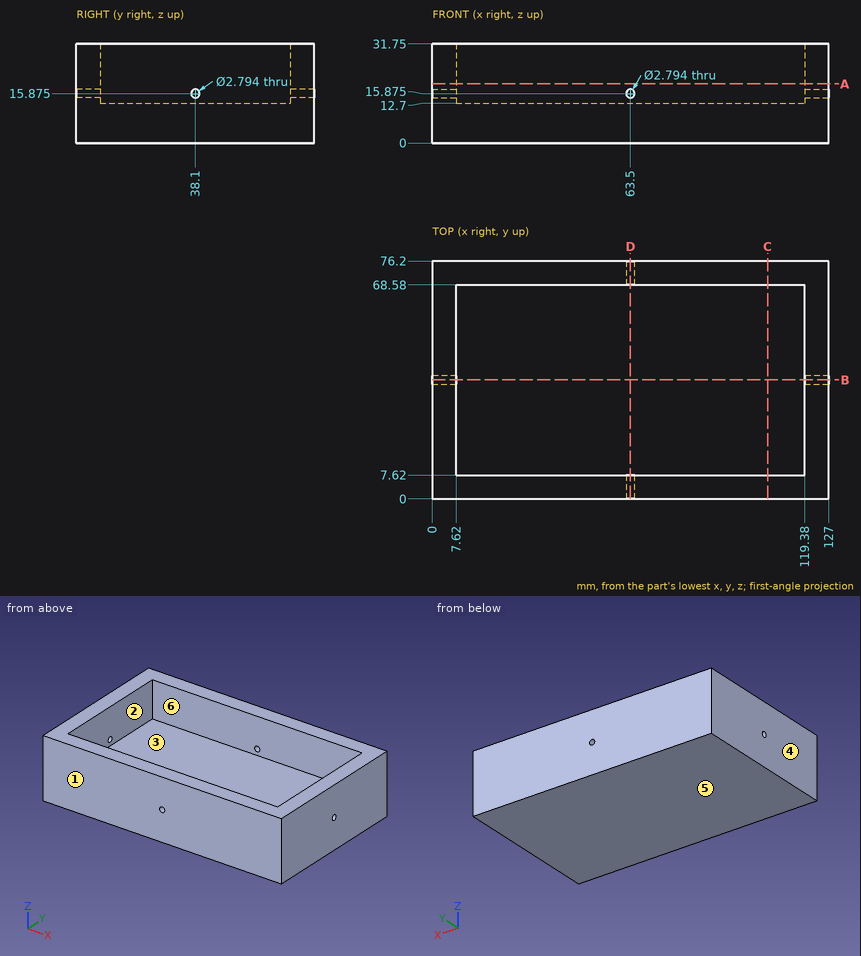
Source: three-view drawing plus pictorial views. Frame: mm from the lowest corner of the part. A direction names the side the tool comes from. Round coordinates to 2 decimals unless told otherwise and drop trailing zeros. Order: outer loops, then holes, each group sorted by start corner. A loop starts at its lowest first (then second) coordinate and runs counter-clockwise, first axis right, second up. Notation, with made-up numbers: (-2.75, -36) -> (44.25, -36) arc R22 ccw to (44.25, -27) -> close; hole circle Ø11 at (-16, 51). An arc over 180 degrees is marked (long way). Use one line per item in the form item = value.
(1) Access query for the marked faces 1 and 2. Directions: +Z, -Z, +X, -X, +Y, -Y. A direction counts if a zero-diameter tool reaches every point of the face in a straight line with its end or side. Return the directions, or none.
Results list:
face_1 = +Z, -Z, +X, -X, -Y
face_2 = +Z
(2) Ray query, probe 1 along X at (y, z) = (27, 14.5); probe 2 along Z at (x, y) = (63.5, 5.75); probe 3 along Y at (x, z) = (110, 17.5). Return the intervals inside material, ascending. Write a range as [from, to].
Results list:
probe_1 = [0, 7.62], [119.38, 127]
probe_2 = [0, 14.48], [17.27, 31.75]
probe_3 = [0, 7.62], [68.58, 76.2]
(3) First-contact query: pin 1 Ø18.5 at (x, y) = (74.5, 39) entering from +Z. Flat tip, straight axial feed; report the tip coordinate or a pass-through.
Results list:
pin_1 = 12.7
(4) Section A-A on z = 19. Return loops of the section in (x, y).
Results list:
outline = (0, 0) -> (127, 0) -> (127, 76.2) -> (0, 76.2) -> close; hole (7.62, 7.62) -> (119.38, 7.62) -> (119.38, 68.58) -> (7.62, 68.58) -> close
(5) Section C-C on x = 107.5. Return loops of the section in (y, z).
Results list:
outline = (0, 0) -> (76.2, 0) -> (76.2, 31.75) -> (68.58, 31.75) -> (68.58, 12.7) -> (7.62, 12.7) -> (7.62, 31.75) -> (0, 31.75) -> close
(6) Draft query along X for the marked faces 3, 4, 5 and 6. Return one class per face: pulls with the +X half, pulls with the -X half, needs draft (parallel to the pull), parting line crosses it, or undercut.
Results list:
face_3 = undercut
face_4 = pulls with the -X half
face_5 = needs draft
face_6 = undercut
(7) Section B-B on y = 38.1. Return loops of the section in (x, z), and give its area (3 significant figures).
Results list:
outline = (0, 0) -> (127, 0) -> (127, 14.48) -> (119.38, 14.48) -> (119.38, 12.7) -> (7.62, 12.7) -> (7.62, 14.48) -> (0, 14.48) -> close; (0, 17.27) -> (7.62, 17.27) -> (7.62, 31.75) -> (0, 31.75) -> close; (119.38, 17.27) -> (127, 17.27) -> (127, 31.75) -> (119.38, 31.75) -> close
area = 1,860 mm^2
(8) Section D-D on x = 63.5. Return loops of the section in (y, z).
Results list:
outline = (0, 0) -> (76.2, 0) -> (76.2, 14.48) -> (68.58, 14.48) -> (68.58, 12.7) -> (7.62, 12.7) -> (7.62, 14.48) -> (0, 14.48) -> close; (0, 17.27) -> (7.62, 17.27) -> (7.62, 31.75) -> (0, 31.75) -> close; (68.58, 17.27) -> (76.2, 17.27) -> (76.2, 31.75) -> (68.58, 31.75) -> close
